Read the model definition and answer for the solid it produces. Units are mm, in the model's axes. A direction names the side the tool comes from. Coordinates: 2 decimals unless noted, no trailing zeros. Write each loop counter-clockwise with the first axis right and the second up, starting at its lowest first coordinate (ties: lowest second). Pieces come first, ordered by that corner, then holes. Notation, with made-up numbers: (26, 60) -> (82, 60) arc R22 cw to (82, 77) -> close; hole circle Ø6 at (-0.5, 55). An arc over 180 degrees is marked (long way). Answer as a JSON object with one key per item and string values. Group by question number.
(1) Find section A-A (z = 6.25). Give the vertices of the cut face in (x, y) (3 decimals), then the cut area to 3 significant figures.
(2) For a pull along X with two mould halves and no side action, classify faces 4 (the face through (-31.25, 316.47, 8.4)), 5 (the face through (-18.6, 337.14, 16.38)), 6 (the face through (-19.81, 337.71, 13.47)) as +X half, -X half, draft (parallel to the pull), parting line (faces both ways), or undercut.
(3) Which of the six approach directions +Z, -Z, +X, -X, +Y, -Y give full straight-line access (tool end or side, diameter ignored) to faces 1 (the face through (-43.535, 331.599, 0.507)), 2 (the face through (-19.028, 332, 8)), 3 (the face through (-19.52, 331.67, 0.51))?
(4) Flat-ended cylindrical pins translate along their axes: P1, Ø1.5, axis at y = 333, z = 3.5, coming from the +X side; P2, Ø10, axis at y = 325.5, z = 9.5, coming from the -X side; P3, Ø2.5, axis at x = -43.28, z = 3.25, coming from the -Y side. Find the tip coordinate at first contact, or state that the pin passes through.
(5) Straight lines are drawn through the part: L1, parallel to X at y = 342.75, z = 13.75; L2, parallel to Y at x = -31.5, z = 12.75; L3, parallel to Y at x = -34.5, z = 16. For each, find the intervals that lie inside material, in ascending order.
(6) Find section B-B (y = 342). Give the vertices of the cut face in (x, z).
from build123d import *

# Parameters (mm, degrees)
SKETCH_1_R             = 9
EXTRUDE_2_DEPTH        = 17
FILLET_7_R             = 5
CHAMFER_3_SIZE         = 1
CHAMFER_4_SIZE         = 1
CHAMFER_5_SIZE         = 0.5
FILLET_9_R             = 2
HOLE_WIZARD_M4_3_D     = 3.3
HOLE_WIZARD_M4_3_DEPTH = 10.1
HOLE_WIZARD_M4_3_TIP   = 0.991420021
HOLE_WIZARD_M4_4_D     = 3.3
HOLE_WIZARD_M4_4_DEPTH = 8
HOLE_WIZARD_M4_4_TIP   = 0.991420021


with BuildPart() as part:
    # 草图1 → 凸台-拉伸2 (new body)
    with BuildSketch(Plane.XY):
        with BuildLine():
            Line((-16.527519938, 348.633233256), (-16.527519938, 338.633233256))
            Line((-16.527519938, 338.633233256), (-19.027519938, 338.633233256))
            Line((-19.027519938, 338.633233256), (-19.027519938, 328.968626967))
            ThreePointArc((-19.027519938, 328.968626967), (-31.527519938, 316.468626967), (-44.027519938, 328.968626967))
            Line((-44.027519938, 328.968626967), (-44.027519938, 338.633233256))
            Line((-44.027519938, 338.633233256), (-46.527519938, 338.633233256))
            Line((-46.527519938, 338.633233256), (-46.527519938, 348.633233256))
            Line((-46.527519938, 348.633233256), (-16.527519938, 348.633233256))
        make_face()
        with Locations((-31.527519938, 328.968626967)):
            Circle(SKETCH_1_R, mode=Mode.SUBTRACT)
    extrude(amount=EXTRUDE_2_DEPTH)

    # 圆角7
    # the kernel refuses this fillet: 5 mm, written as the material it adds along each edge
    with BuildSketch(Plane(origin=(-19.027519938, 338.633233256, 0), x_dir=(1, 0, 0), z_dir=(0, 0, 1))) as fillet_7_piece_1:
        with BuildLine():
            CenterArc((5, -4.330127019), FILLET_7_R, 120, 60)
            Line((0, -4.330127019), (-0.1, -4.330127019))
            Line((-0.1, -4.330127019), (-0.1, 0))
            Line((-0.1, 0), (0, 0.1))
            ThreePointArc((0, 0.1), (1.25, 0.1), (2.45, 0.08660254))
            Line((2.45, 0.08660254), (2.5, 0))
        make_face()
    extrude(amount=17)
    with BuildSketch(Plane(origin=(-44.027519938, 338.633233256, 0), x_dir=(0, -1, 0), z_dir=(0, 0, 1))) as fillet_7_piece_2:
        with BuildLine():
            CenterArc((4.330127019, -5), FILLET_7_R, 90, 60)
            Line((0, -2.5), (-0.08660254, -2.45))
            ThreePointArc((-0.08660254, -2.45), (-0.1, -1.25), (-0.1, 0))
            Line((-0.1, 0), (0, 0.1))
            Line((0, 0.1), (4.330127019, 0.1))
            Line((4.330127019, 0.1), (4.330127019, 0))
        make_face()
    extrude(amount=17)

    # 倒角3
    chamfer_3_edges = [part.edges().sort_by_distance(p)[0] for p in [
        (-31.527519938, 316.468626967, 17),
        (-19.027519938, 331.635866602, 17),
        (-44.027519938, 331.635866602, 17),
        (-18.357646957, 336.803106237, 17),
        (-44.697392919, 336.803106237, 17),
    ]]
    chamfer(chamfer_3_edges, length=CHAMFER_3_SIZE)

    # 倒角4
    chamfer_4_edges = [part.edges().sort_by_distance(p)[0] for p in [
        (-19.027519938, 331.635866602, 0),
        (-31.527519938, 316.468626967, 0),
        (-40.527519938, 328.968626967, 0),
        (-40.527519938, 328.968626967, 17),
        (-44.027519938, 331.635866602, 0),
        (-18.357646957, 336.803106237, 0),
        (-44.697392919, 336.803106237, 0),
    ]]
    chamfer(chamfer_4_edges, length=CHAMFER_4_SIZE)

    # 倒角5
    chamfer_5_edges = [part.edges().sort_by_distance(p)[0] for p in [
        (-16.527519938, 344.195347776, 0),
        (-16.527519938, 344.195347776, 17),
        (-46.527519938, 344.195347776, 0),
        (-46.527519938, 344.195347776, 17),
    ]]
    chamfer(chamfer_5_edges, length=CHAMFER_5_SIZE)

    # 圆角9
    fillet_9_edges = [part.edges().sort_by_distance(p)[0] for p in [
        (-16.527519938, 338.633233256, 8.5),
        (-46.527519938, 338.633233256, 8.5),
    ]]
    fillet(fillet_9_edges, radius=FILLET_9_R)

    # M4 螺纹孔3
    with Locations(Plane(origin=(0, 348.633233256, 0), x_dir=(1, 0, 0), z_dir=(0, 1, 0))):
        with Locations((-19.777519938, -13.75), (-43.277519938, -13.75), (-43.277519938, -3.248268424), (-19.777519938, -3.248268424)):
            Hole(HOLE_WIZARD_M4_3_D / 2, depth=HOLE_WIZARD_M4_3_DEPTH)
            with Locations((0, 0, -(HOLE_WIZARD_M4_3_DEPTH + HOLE_WIZARD_M4_3_TIP / 2))):  # 118° drill point
                Cone(0, HOLE_WIZARD_M4_3_D / 2, HOLE_WIZARD_M4_3_TIP, mode=Mode.SUBTRACT)

    # M4 螺纹孔4
    with Locations(Plane(origin=(0, 348.633233256, 0), x_dir=(1, 0, 0), z_dir=(0, 1, 0))):
        with Locations((-37.241924816, -8.499134212), (-25.81311506, -8.499134212)):
            Hole(HOLE_WIZARD_M4_4_D / 2, depth=HOLE_WIZARD_M4_4_DEPTH)
            with Locations((0, 0, -(HOLE_WIZARD_M4_4_DEPTH + HOLE_WIZARD_M4_4_TIP / 2))):  # 118° drill point
                Cone(0, HOLE_WIZARD_M4_4_D / 2, HOLE_WIZARD_M4_4_TIP, mode=Mode.SUBTRACT)


solid = part.part
Results below:
{
 "1": {"outline": "(-46.528, 339.665) arc R2 ccw to (-45.813, 338.133) arc R5 cw to (-44.028, 334.303) -> (-44.028, 328.969) arc R12.5 ccw to (-19.028, 328.969) -> (-19.028, 334.303) arc R5 cw to (-17.242, 338.133) arc R2 ccw to (-16.528, 339.665) -> (-16.528, 348.633) -> (-46.528, 348.633) -> close; hole circle Ø18 at (-31.528, 328.969)", "area": "539 mm2"},
 "2": {"face 4": "parting line", "face 5": "+X half", "face 6": "undercut"},
 "3": {"face 1": "-Z, -X, -Y", "face 2": "+Z, -Z, +X, -Y", "face 3": "-Z, +X, -Y"},
 "4": {"P1": "stops at x = -19.03", "P2": "stops at x = -44.03", "P3": "stops at y = 322.19"},
 "5": {"L1": "x = -46.53 to -44.93, -41.63 to -21.43, -18.13 to -16.53", "L2": "y = 316.47 to 319.97, 337.97 to 348.63", "L3": "y = 316.83 to 320.47, 337.46 to 348.63"},
 "6": {"outline": "(-46.53, 0.5) -> (-46.03, 0) -> (-17.03, 0) -> (-16.53, 0.5) -> (-16.53, 16.5) -> (-17.03, 17) -> (-46.03, 17) -> (-46.53, 16.5) -> close; hole circle Ø3.3 at (-43.28, 3.25); hole circle Ø3.3 at (-43.28, 13.75); hole circle Ø3.3 at (-37.24, 8.5); hole circle Ø3.3 at (-25.81, 8.5); hole circle Ø3.3 at (-19.78, 3.25); hole circle Ø3.3 at (-19.78, 13.75)"}
}
